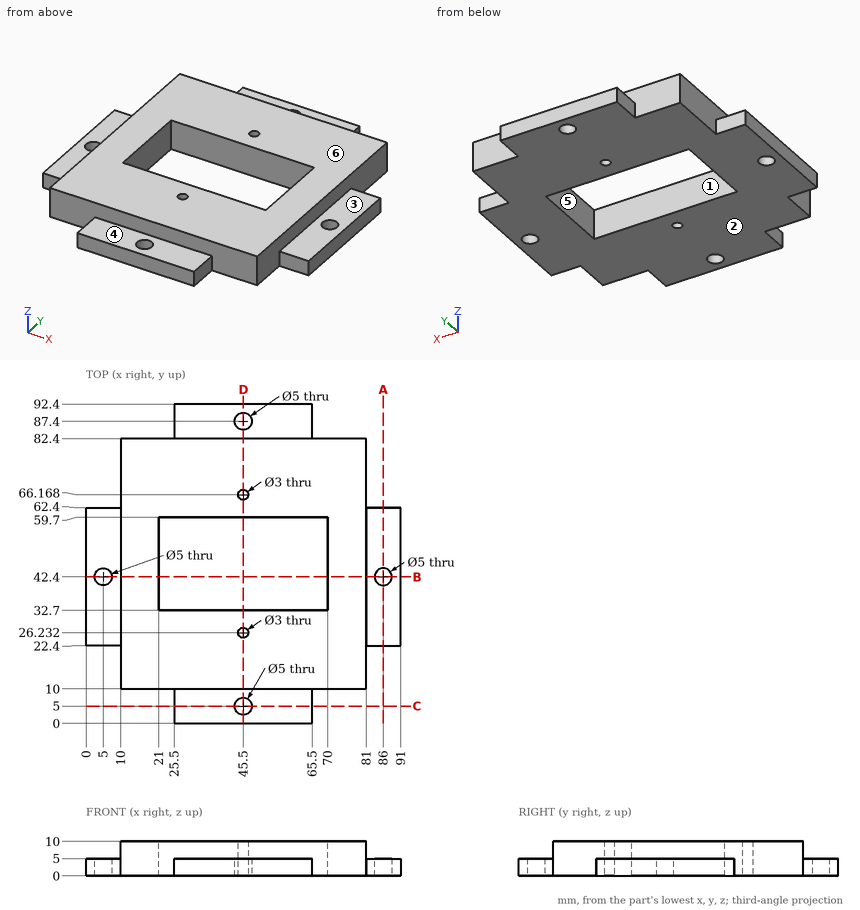
Print and shaded views of the part. All mm, measured from the part's lowest x, y and z. A direction names the side the tool comes from. Give positions to 0.01 mm unless a question says otherwise; leave off trailing zeros. Order: outer loops, then holes, each group sorted by start corner. A loop starts at its lowest first (then second) coordinate and runs counter-clockwise, first axis right, second up. Notation, with made-up numbers: (39, 0.5) - (57, 0.5) arc R9 ccw to (57, 7.5) - close; hole circle Ø4 at (43, 55). An arc over 180 degrees is marked (long way). One line per item, written item: value.
Item 1: Slice it at C-C (y = 5). List the corners of the cut face in (x, z).
Response values:
outline: (25.5, 0) - (43, 0) - (43, 5) - (25.5, 5) - close; (48, 0) - (65.5, 0) - (65.5, 5) - (48, 5) - close
Item 2: Two-plate mould, pull along X, no slides. Class the marked faces 5 and 6: released by +X, released by -X, zero draft, split by the parting line, or undercut.
Response values:
face 5: undercut
face 6: zero draft
Item 3: Pin check, flat tips, straight feed: pin 1 Ø8 at (x, y) = (5, 42.4) entering from +Z; pin 2 Ø1.5 at (y, z) = (7, 2.5) entering from +X; pin 3 Ø5.5 at (x, z) = (88, 3) entering from -Y. Stop position of each tip, or through.
Response values:
pin 1: z = 5
pin 2: x = 65.5
pin 3: y = 22.4
Item 4: Slice it at D-D (x = 45.5). List the corners of the cut face in (y, z).
Response values:
outline: (0, 0) - (2.5, 0) - (2.5, 5) - (0, 5) - close; (7.5, 0) - (24.73, 0) - (24.73, 10) - (10, 10) - (10, 5) - (7.5, 5) - close; (27.73, 0) - (32.7, 0) - (32.7, 10) - (27.73, 10) - close; (59.7, 0) - (64.67, 0) - (64.67, 10) - (59.7, 10) - close; (67.67, 0) - (84.9, 0) - (84.9, 5) - (82.4, 5) - (82.4, 10) - (67.67, 10) - close; (89.9, 0) - (92.4, 0) - (92.4, 5) - (89.9, 5) - close
Item 5: Tool access for the marked faces 1, 2, 3 and 4: list every direction of +Z, -Z, +X, -X, +Y, -Y with a clear straight run to the whole face (end or side of a thin tool).
Response values:
face 1: +Z, -Z
face 2: -Z, +X, -X, +Y, -Y
face 3: +Z, +X, +Y, -Y
face 4: +Z, +X, -X, -Y
Item 6: Slice it at B-B (y = 42.4). List the corners of the cut face in (x, z), then the cut area to 3 significant figures.
Response values:
outline: (0, 0) - (2.5, 0) - (2.5, 5) - (0, 5) - close; (7.5, 0) - (21, 0) - (21, 10) - (10, 10) - (10, 5) - (7.5, 5) - close; (70, 0) - (83.5, 0) - (83.5, 5) - (81, 5) - (81, 10) - (70, 10) - close; (88.5, 0) - (91, 0) - (91, 5) - (88.5, 5) - close
area: 270 mm2
Item 7: Slice it at A-A (x = 86). List the corners of the cut face in (y, z).
Response values:
outline: (22.4, 0) - (39.9, 0) - (39.9, 5) - (22.4, 5) - close; (44.9, 0) - (62.4, 0) - (62.4, 5) - (44.9, 5) - close
Item 8: Wall check: line 1 (Y direction, x = 22.5, z = 6); line 2 (X direction, y = 39, z = 6.25); line 3 (Y direction, x = 46.5, z = 7.75). Give the ranges that are in metal, low to high.
Response values:
line 1: 10 to 32.7, 59.7 to 82.4
line 2: 10 to 21, 70 to 81
line 3: 10 to 25.11, 27.35 to 32.7, 59.7 to 65.05, 67.29 to 82.4
